Geometry check sheet. Reference: the model listing, model coordinates, mm. Give positions to 0.01 mm unless a question says otherwise; leave off trailing zeros. Order: outer loops, then holes, each group sorted by start corner. A loop starts at its lowest first (then second) coordinate and runs counter-clockwise, first axis right, second up.
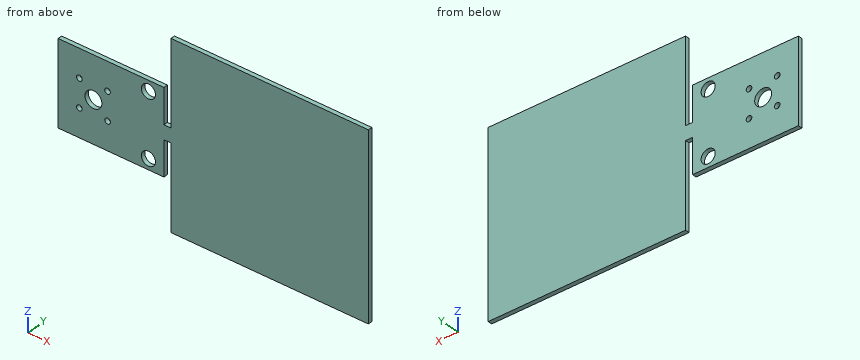
from build123d import *

# Parameters (mm, degrees)
SKETCH1_R             = 6
SKETCH1_R_2           = 2
SKETCH1_R_3           = 7.5
BOSS_EXTRUDE1_DEPTH   = 1.5
SKETCH2_W             = 115.219632385
SKETCH2_H             = 145.344306737
CUT_EXTRUDE1_DEPTH    = 164.505351594
DELETEFACE1_START     = -1.5
DELETEFACE1_OUTLINE_R = 7.5
DELETEFACE1_DEPTH     = 3
SKETCH4_R             = 5
CUT_EXTRUDE2_DEPTH    = 164.505351594


# Read off the part's stored shape, not the designer's step: DeleteFace1
with BuildPart() as part:
    # Sketch1 → Boss-Extrude1 (new, symmetric)
    with BuildSketch(Plane(origin=(0, 0, 0), x_dir=(1, 0, 0), z_dir=(0, 1, 0))):
        Polygon((70, 65), (70, 5), (75, 5), (75, 30), (150, 30), (150, -30), (75, -30), (75, -5), (70, -5), (70, -65), (-70, -65), (-70, -5), (-75, -5), (-75, -30), (-150, -30), (-150, 30), (-75, 30), (-75, 5), (-70, 5), (-70, 65), align=None)
        with Locations(Location((125, 0, 0), (0, 0, 270))):
            Circle(SKETCH1_R, mode=Mode.SUBTRACT)
        with Locations(Location((115, 10, 0), (0, 0, 270))):
            Circle(SKETCH1_R_2, mode=Mode.SUBTRACT)
        with Locations(Location((135, 10, 0), (0, 0, 90))):
            Circle(SKETCH1_R_2, mode=Mode.SUBTRACT)
        with Locations(Location((135, -10, 0), (0, 0, 270))):
            Circle(SKETCH1_R_2, mode=Mode.SUBTRACT)
        with Locations(Location((115, -10, 0), (0, 0, 90))):
            Circle(SKETCH1_R_2, mode=Mode.SUBTRACT)
        with Locations(Location((-115, -10, 0), (0, 0, 270))):
            Circle(SKETCH1_R_2, mode=Mode.SUBTRACT)
        with Locations(Location((-135, -10, 0), (0, 0, 90))):
            Circle(SKETCH1_R_2, mode=Mode.SUBTRACT)
        with Locations(Location((-135, 10, 0), (0, 0, 270))):
            Circle(SKETCH1_R_2, mode=Mode.SUBTRACT)
        with Locations(Location((-125, 0, 0), (0, 0, 90))):
            Circle(SKETCH1_R, mode=Mode.SUBTRACT)
        with Locations(Location((-115, 10, 0), (0, 0, 90))):
            Circle(SKETCH1_R_2, mode=Mode.SUBTRACT)
        with Locations(Location((100, 0, 0), (0, 0, 270))):
            Circle(SKETCH1_R_3, mode=Mode.SUBTRACT)
        with Locations(Location((-100, 0, 0), (0, 0, 90))):
            Circle(SKETCH1_R_3, mode=Mode.SUBTRACT)
    extrude(amount=BOSS_EXTRUDE1_DEPTH, both=True)

    # Sketch2 → Cut-Extrude1 (cut, through all)
    with BuildSketch(Plane(origin=(0, 1.5, 0), x_dir=(1, 0, 0), z_dir=(0, 1, 0))):
        with Locations((127.609816193, -7.672153369)):
            Rectangle(SKETCH2_W, SKETCH2_H)
    extrude(amount=-CUT_EXTRUDE1_DEPTH, mode=Mode.SUBTRACT)

    # DeleteFace1 outline → DeleteFace1 (add)
    with BuildSketch(Plane(origin=(0, 0, 0), x_dir=(1, 0, 0), z_dir=(0, 1, 0)).offset(DELETEFACE1_START)):
        with Locations((-100, 0)):
            Circle(DELETEFACE1_OUTLINE_R)
    extrude(amount=DELETEFACE1_DEPTH)

    # Sketch4 → Cut-Extrude2 (cut, through all)
    with BuildSketch(Plane(origin=(0, 1.5, 0), x_dir=(1, 0, 0), z_dir=(0, 1, 0))):
        with Locations(Location((-86.02885683, -22.5, 0), (0, 0, 270))):
            Circle(SKETCH4_R)
        with Locations(Location((-86.02885683, 22.5, 0), (0, 0, 90))):
            Circle(SKETCH4_R)
    extrude(amount=-CUT_EXTRUDE2_DEPTH, mode=Mode.SUBTRACT)


solid = part.part
Item 1: Scan lines: L1, parallel to Z at x = -135, y = -0.5; L2, parallel to X at y = -0.4, z = 10; L3, parallel to X at y = -0.6, z = 22.5. Record each from-to range of solid material in increasing order.
Reported:
L1: z = -30 to -12, -8 to 8, 12 to 30
L2: x = -150 to -137, -133 to -117, -113 to -75, -70 to 70
L3: x = -150 to -91.03, -81.03 to -75, -70 to 70
Item 2: Sectioned sample at B-B (x = -125). Enter the section's corners in (y, z).
Reported:
outline: (-1.5, -30) - (1.5, -30) - (1.5, -6) - (-1.5, -6) - close; (-1.5, 6) - (1.5, 6) - (1.5, 30) - (-1.5, 30) - close
Item 3: Sectioned sample at C-C (z = 22.5). Enter the section's corners in (x, y), and give its area (3 significant figures).
Reported:
outline: (-150, -1.5) - (-91.03, -1.5) - (-91.03, 1.5) - (-150, 1.5) - close; (-81.03, -1.5) - (-75, -1.5) - (-75, 1.5) - (-81.03, 1.5) - close; (-70, -1.5) - (70, -1.5) - (70, 1.5) - (-70, 1.5) - close
area: 615 mm2
Item 4: Sectioned sample at D-D (y = -0.3). Enter the section's corners in (x, z), and give its area (3 significant figures).
Reported:
outline: (-150, -30) - (-75, -30) - (-75, -5) - (-70, -5) - (-70, -65) - (70, -65) - (70, 65) - (-70, 65) - (-70, 5) - (-75, 5) - (-75, 30) - (-150, 30) - close; hole circle Ø4 at (-135, -10); hole circle Ø4 at (-135, 10); hole circle Ø12 at (-125, 0); hole circle Ø4 at (-115, -10); hole circle Ø4 at (-115, 10); hole circle Ø10 at (-86.03, -22.5); hole circle Ø10 at (-86.03, 22.5)
area: 22,400 mm2
Item 5: Gauge pin test, flat ends, axial feed: pin 1 (1.5 mm diameter, centred on x = -73, y = -0.5, fed in from -Z); pin 2 (3 mm diameter, centred on x = -115, z = 10, fed in from +Y). Record the tip position at first contact, or that the pin passes through.
Reported:
pin 1: stops at z = -5
pin 2: passes through
Item 6: Sectioned sample at A-A (z = 0). Enter the section's corners in (x, y), and give its area (3 significant figures).
Reported:
outline: (-150, -1.5) - (-131, -1.5) - (-131, 1.5) - (-150, 1.5) - close; (-119, -1.5) - (70, -1.5) - (70, 1.5) - (-119, 1.5) - close
area: 624 mm2
